Read the model definition and answer for the solid it produces. Units are mm, in the model's axes. A direction names the side the tool comes from. Give positions to 0.01 mm unless a question says otherwise; leave off trailing zeros. Loops run counter-clockwise (first coordinate to the right, second up) from the corner with the lowest first, then second, coordinate; pieces in that order, holes last. Notation, with made-up numbers: (-34.75, 18) - (-29.75, 18) arc R19 ccw to (-29.75, 28) - close; hole circle Ø9 at (-22.5, -38). An arc over 180 degrees is marked (long way). Write item = value, one per line.
```python
from build123d import *

# Parameters (mm, degrees)
EXTRUDE_1_DEPTH     = 15
CHAMFER_1_SIZE      = 4
SKETCH_3_OUTSIDE_W  = 123.748
SKETCH_3_OUTSIDE_H  = 63.748
SKETCH_3_OUTSIDE_R  = 20
CUT_EXTRUDE_1_DEPTH = 8
SKETCH_4_R          = 5
EXTRUDE_2_DEPTH     = 14


with BuildPart() as part:
    # 草图1 → 凸台-拉伸1 (new body)
    with BuildSketch(Plane(origin=(0, 0, 0), x_dir=(1, 0, 0), z_dir=(0, 1, 0))):
        with BuildLine():
            Line((30, -20), (-30, -20))
            ThreePointArc((-30, -20), (-50, 0), (-30, 20))
            Line((-30, 20), (30, 20))
            ThreePointArc((30, 20), (50, 0), (30, -20))
        make_face()
    extrude(amount=EXTRUDE_1_DEPTH)

    # 倒角1
    chamfer_1_edges = [part.edges().sort_by_distance(p)[0] for p in [
        (-50, 15, 0),
        (0, 15, 20),
        (50, 15, 0),
        (0, 15, -20),
    ]]
    chamfer(chamfer_1_edges, length=CHAMFER_1_SIZE)

    # 草图3 outside → 切除-拉伸1 (cut)
    with BuildSketch(Plane.XZ):
        Rectangle(SKETCH_3_OUTSIDE_W, SKETCH_3_OUTSIDE_H)
        with Locations(Location((-30, 0, 0), (0, 0, 90))):
            Circle(SKETCH_3_OUTSIDE_R, mode=Mode.SUBTRACT)
        with Locations(Location((30, 0, 0), (0, 0, 90))):
            Circle(SKETCH_3_OUTSIDE_R, mode=Mode.SUBTRACT)
    extrude(amount=-CUT_EXTRUDE_1_DEPTH, mode=Mode.SUBTRACT)

    # 草图4 → 凸台-拉伸2 (add)
    with BuildSketch(Plane.XZ.offset(-8)):
        with Locations(Location((0, 0, 0), (0, 0, 270))):
            Circle(SKETCH_4_R)
    extrude(amount=EXTRUDE_2_DEPTH)


solid = part.part
```
1) Find the intervals of material crossed by probe 1 along Y at (x, z) = (14, 14); probe 2 along Y at (x, z) = (15, 0); probe 3 along X at (y, z) = (7.25, 7) (3 decimals), in increasing order.
Output:
probe_1 = 8 to 15
probe_2 = 0 to 15
probe_3 = -48.735 to -11.265, 11.265 to 48.735
2) A cutting plane is placed at B-B on x = 0. Determine the outline of the cut face in (y, z).
Output:
outline = (-6, -5) - (8, -5) - (8, -20) - (11, -20) - (15, -16) - (15, 16) - (11, 20) - (8, 20) - (8, 5) - (-6, 5) - close
3) A tool of negligible diameter and unlimited length cuts with its end or side. For faces 1 (the face through (30, 0, 0)), 2 (the face through (49.83, 5.42, 2.6)), 3 (the face through (0, 13, -18)), from which of +Z, -Z, +X, -X, +Y, -Y can it reach the whole face along a straight path? Write none if from no direction.
Output:
face_1 = +Z, -Z, +X, -Y
face_2 = -Y
face_3 = -Z, +X, -X, +Y
4) Each of these flat-tipped pins is pushed along its axis until it touches: P1, Ø6, axis at y = 4.5, z = 14, coming from the +X side; P2, Ø3, axis at x = 26.5, z = -11.5, coming from the -Y side; P3, Ø8, axis at y = -0.5, z = 14.5, coming from the -X side. Where does it stop, or does it pass through?
Output:
P1 = 46.7
P2 = 0
P3 = -47
5) A cutting plane is placed at C-C on y = -1. Determine the outline of the cut face in (x, z).
Output:
outline = circle Ø10 at (0, 0)
6) The mould has two halves that part along X. Classify faces 4 (the face through (-30, 0, 0)), 5 (the face through (6, 8, 0)), 6 (the face through (46.19, 14.806, -0.356)), 7 (the face through (-4.88, 1.1, 1.08)): pulls with the +X half, pulls with the -X half, needs draft (parallel to the pull), parting line crosses it, or undercut.
Output:
face_4 = needs draft
face_5 = undercut
face_6 = pulls with the +X half
face_7 = undercut
7) A cutting plane is placed at A-A on z = 0. Determine the outline of the cut face in (x, y), then the cut area to 3 significant figures.
Output:
outline = (-50, 0) - (-10, 0) - (-10, 8) - (-5, 8) - (-5, -6) - (5, -6) - (5, 8) - (10, 8) - (10, 0) - (50, 0) - (50, 11) - (46, 15) - (-46, 15) - (-50, 11) - close
area = 1,460 mm²
